The model under review builds one solid part; all positions refer to its coordinate system, in mm. A direction names the side the tool comes from. Coordinates: 2 decimals unless noted, no trailing zeros. Use a Markdown table: item, result. Add a question column.
1) To check wall thickness, follow L1, parallel to X at y = -88.5, z = -2.5; L2, parallel to X at y = 34, z = 2.5; L3, parallel to Y at x = -28.5, z = -0.75. State the ranges of each line that lie inside material, in increasing order. Write a range as [from, to].
2) Clearance check with flat-ended pins moving along their axes: pin 1 (6 mm diameter, centred on x = 47.5, z = 3.5, fed in from +Y); pin 2 (6 mm diameter, centred on x = 21.5, z = 1.5, fed in from -Y); pin 3 (1.1 mm diameter, centred on x = 74.5, y = 43.5, fed in from -Z). State where each tip first meets the part, or that it passes through.
3) The part is to be moulded in two halves that separate along Y. For faces 1 (the flat face through (-87.43, -89.06, -1.9)), 2 (the conical face through (89.57, 99.68, -1.9)), 3 (the conical face through (1, -37.9, -1.7)), 4 (the cylindrical face through (76.91, 41.25, 4.15)), say which applies: pulls with the +Y half, pulls with the -Y half, needs draft (parallel to the pull), parting line crosses it, or undercut.
4) For faces 5 (the flat face through (78.3, 42, -1.9)), 6 (the flat face through (-123, -129, -5)), 7 (the flat face through (92.788, 83.125, 3.689)), 8 (the flat face through (72.804, 33.728, -1.718)), list the 3-axis set-ups (+Z, -Z, +X, -X, +Y, -Y) from which the entire face can be reached by the end or side of a thin tool; tool diameter is ignored.
```python
from build123d import *

# Parameters (mm, degrees)
EXTRUSION2_DEPTH        = 11.2
EXTRUSION2_DRAFT        = -4
COQUE1_T                = -1.5
CONG_1_R                = 2
ESQUISSE4_R             = 12.5
ENL_V_MAT_EXTRU_1_DEPTH = 190.035497549
EXTRUSION3_START        = -1.5
EXTRUSION3_DEPTH        = 1.5
EXTRUSION4_DEPTH        = 1
EXTRUSION5_DEPTH        = 1


with BuildPart() as part:
    # Esquisse3 → Extrusion2 (with draft: the straight prism first)
    with BuildSketch(Plane(origin=(0, 0, -6.5), x_dir=(-1, 0, 0), z_dir=(0, 0, -1))):
        with BuildLine():
            Line((-34.418091678, 13.052373199), (-71.398662192, 93.016853596))
            ThreePointArc((-71.398662192, 93.016853596), (-89.98211464, 99.847321744), (-96.812582788, 81.263869296))
            Line((-96.812582788, 81.263869296), (-59.832012274, 1.299388899))
            ThreePointArc((-59.832012274, 1.299388899), (-20.171981407, -55.724047413), (36.599420799, -95.744020285))
            Line((36.599420799, -95.744020285), (113.622178214, -131.957364461))
            ThreePointArc((113.622178214, -131.957364461), (132.248468989, -125.244593651), (125.535698179, -106.618302875))
            Line((125.535698179, -106.618302875), (48.512940764, -70.4049587))
            ThreePointArc((48.512940764, -70.4049587), (-0.310465133, -35.987782029), (-34.418091678, 13.052373199))
        make_face()
    extrude(amount=-EXTRUSION2_DEPTH)
    # Extrusion2: the draft: its side faces are tilted about the plane it starts from
    extrusion2_sides = [part.faces().sort_by_distance(p)[0] for p in [
        (52.908376935, 53.034613397, -0.9),
        (89.98211464, 99.847321744, -0.9),
        (78.322297531, 41.281629097, -0.9),
        (20.171981407, -55.724047413, -0.9),
        (-75.110799506, -113.850692373, -0.9),
        (-132.248468989, -125.244593651, -0.9),
        (-87.024319472, -88.511630788, -0.9),
        (0.310465133, -35.987782029, -0.9),
    ]]
    draft(extrusion2_sides, Plane(origin=(0, 0, -6.5), x_dir=(-1, 0, 0), z_dir=(0, 0, -1)), EXTRUSION2_DRAFT)

    # Coque1
    coque1_openings = [part.faces().sort_by_distance(p)[0] for p in [
        (55.899933032, 51.651130998, -6.5),
    ]]
    offset(amount=COQUE1_T, openings=coque1_openings, kind=Kind.INTERSECTION)

    # Congé1
    cong_1_edges = [part.edges().sort_by_distance(p)[0] for p in [
        (89.653375151, 99.136475965, 4.7),
        (77.611451752, 41.610368587, 4.7),
        (19.616440402, -55.172009765, 4.7),
        (-75.444029294, -113.141940455, 4.7),
        (-131.539717071, -124.911363863, 4.7),
        (-86.691089684, -89.220382705, 4.7),
        (0.866006138, -36.539819677, 4.7),
        (53.619222714, 52.705873908, 4.7),
    ]]
    fillet(cong_1_edges, radius=CONG_1_R)

    # Esquisse4 → Enlèv. mat.-Extru.1 (cut, through all)
    with BuildSketch(Plane.XY.offset(4.7)):
        with Locations(Location((-119.578938197, -119.287833668, 0), (0, 0, 319.931231963))):
            Circle(ESQUISSE4_R)
        with BuildLine():
            Line((88.428033532, 98.869247275), (85.254326361, 92.00662073))
            ThreePointArc((85.254326361, 92.00662073), (81.917712078, 91.636253796), (79.567422384, 89.239108642))
            Line((79.567422384, 89.239108642), (72.760122224, 92.387229437))
            ThreePointArc((72.760122224, 92.387229437), (79.327015541, 98.690898906), (88.428033532, 98.869247275))
        make_face()
        with BuildLine():
            Line((90.243313574, 98.029748396), (87.069606403, 91.167121851))
            ThreePointArc((87.069606403, 91.167121851), (88.948261451, 88.384888621), (88.643822596, 85.041614249))
            Line((88.643822596, 85.041614249), (95.451122756, 81.893493455))
            ThreePointArc((95.451122756, 81.893493455), (96.001427458, 90.979609311), (90.243313574, 98.029748396))
        make_face()
    extrude(amount=-ENL_V_MAT_EXTRU_1_DEPTH, mode=Mode.SUBTRACT)

    # Esquisse5 → Extrusion3 (add)
    with BuildSketch(Plane(origin=(0, 0, -6.5), x_dir=(-1, 0, 0), z_dir=(0, 0, -1)).offset(EXTRUSION3_START)):
        with BuildLine():
            Line((127.456927912, -109.582820632), (125.904179404, -112.885386975))
            ThreePointArc((125.904179404, -112.885386975), (128.045865957, -116.236418537), (128.534282025, -120.183275965))
            Line((128.534282025, -120.183275965), (131.836848368, -121.736024473))
            ThreePointArc((131.836848368, -121.736024473), (131.338560086, -115.049757096), (127.456927912, -109.582820632))
        make_face()
        with BuildLine():
            Line((125.98138489, -125.613074876), (129.283951233, -127.165823384))
            ThreePointArc((129.283951233, -127.165823384), (123.817014768, -131.047455557), (117.130747392, -131.54574384))
            Line((117.130747392, -131.54574384), (118.6834959, -128.243177497))
            ThreePointArc((118.6834959, -128.243177497), (122.630353328, -127.754761428), (125.98138489, -125.613074876))
        make_face()
    extrude(amount=EXTRUSION3_DEPTH)

    # Esquisse6 → Extrusion4 (add)
    with BuildSketch(Plane(origin=(-86.746444122, -89.10264844, 2.839512947), x_dir=(0, 0, -1), z_dir=(0.9049664851912623, 0.42548285591851137, 0))):
        with BuildLine():
            Line((-0.360487053, -4.346917634), (2.339512947, -4.346917634))
            ThreePointArc((2.339512947, -4.346917634), (2.693066338, -4.200471025), (2.839512947, -3.846917634))
            Line((2.839512947, -3.846917634), (2.839512947, -2.846917634))
            ThreePointArc((2.839512947, -2.846917634), (2.985959557, -2.493364244), (3.339512947, -2.346917634))
            Line((3.339512947, -2.346917634), (8.339512947, -2.346917634))
            ThreePointArc((8.339512947, -2.346917634), (8.693066338, -2.200471025), (8.839512947, -1.846917634))
            Line((8.839512947, -1.846917634), (8.839512947, -0.885543888))
            Line((8.839512947, -0.885543888), (-0.360487053, -1.528870557))
            Line((-0.360487053, -1.528870557), (-0.360487053, -4.346917634))
        make_face()
        with BuildLine():
            Line((-0.360487053, -22.346917634), (2.339512947, -22.346917634))
            ThreePointArc((2.339512947, -22.346917634), (2.693066338, -22.493364244), (2.839512947, -22.846917634))
            Line((2.839512947, -22.846917634), (2.839512947, -23.846917634))
            ThreePointArc((2.839512947, -23.846917634), (2.985959557, -24.200471025), (3.339512947, -24.346917634))
            Line((3.339512947, -24.346917634), (8.339512947, -24.346917634))
            ThreePointArc((8.339512947, -24.346917634), (8.693066338, -24.493364244), (8.839512947, -24.846917634))
            Line((8.839512947, -24.846917634), (8.839512947, -25.808291381))
            Line((8.839512947, -25.808291381), (-0.360487053, -25.164964712))
            Line((-0.360487053, -25.164964712), (-0.360487053, -22.346917634))
        make_face()
    extrude(amount=EXTRUSION4_DEPTH)

    # Esquisse7 → Extrusion5 (add)
    with BuildSketch(Plane(origin=(52.908376935, 53.034613397, -6.5), x_dir=(-0.9076400212812858, 0.4197494392712243, 0), z_dir=(0.4197494392712243, 0.9076400212812858, 0))):
        with BuildLine():
            Line((-23, 9.7), (-23, 7))
            ThreePointArc((-23, 7), (-23.146446609, 6.646446609), (-23.5, 6.5))
            Line((-23.5, 6.5), (-24.5, 6.5))
            ThreePointArc((-24.5, 6.5), (-24.853553391, 6.353553391), (-25, 6))
            Line((-25, 6), (-25, 1))
            ThreePointArc((-25, 1), (-25.146446609, 0.646446609), (-25.5, 0.5))
            Line((-25.5, 0.5), (-26.461373747, 0.5))
            Line((-26.461373747, 0.5), (-25.818047077, 9.7))
            Line((-25.818047077, 9.7), (-23, 9.7))
        make_face()
        with BuildLine():
            Line((-5, 9.7), (-5, 7))
            ThreePointArc((-5, 7), (-4.853553391, 6.646446609), (-4.5, 6.5))
            Line((-4.5, 6.5), (-3.5, 6.5))
            ThreePointArc((-3.5, 6.5), (-3.146446609, 6.353553391), (-3, 6))
            Line((-3, 6), (-3, 1))
            ThreePointArc((-3, 1), (-2.853553391, 0.646446609), (-2.5, 0.5))
            Line((-2.5, 0.5), (-1.538626253, 0.5))
            Line((-1.538626253, 0.5), (-2.181952923, 9.7))
            Line((-2.181952923, 9.7), (-5, 9.7))
        make_face()
    extrude(amount=EXTRUSION5_DEPTH)


solid = part.part
```
From the geometry:
| question | item | result |
|---|---|---|
| 1 | L1 | x = [-86.34, -82.81], [-26.3, -23.21] |
| 1 | L2 | x = [44.8, 46.46], [72.6, 74.26] |
| 1 | L3 | y = [-91.26, -89.55], [-61.58, -59.79] |
| 2 | pin 1 | stops at y = 46.14 |
| 2 | pin 2 | stops at y = -56.62 |
| 2 | pin 3 | stops at z = 0 |
| 3 | face 1 | pulls with the +Y half |
| 3 | face 2 | parting line crosses it |
| 3 | face 3 | undercut |
| 3 | face 4 | pulls with the -Y half |
| 4 | face 5 | +Z, +X, -Y |
| 4 | face 6 | +Z |
| 4 | face 7 | +Z, -Z |
| 4 | face 8 | -Z |
